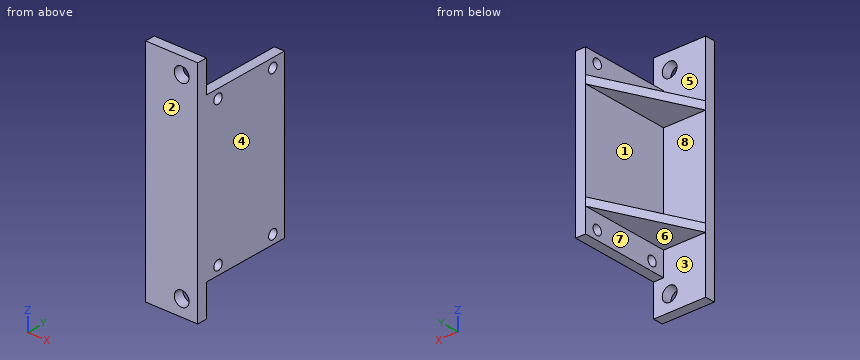
from build123d import *

# Parameters (mm, degrees)
SKETCH1_W           = 16.51
SKETCH1_H           = 71.632288028
SKETCH1_R           = 2.3495
BOSS_EXTRUDE1_DEPTH = 3.175
SKETCH2_W           = 51.312288028
SKETCH2_H           = 28.575
SKETCH2_R           = 1.524
BOSS_EXTRUDE2_DEPTH = 3.175
BOSS_EXTRUDE3_DEPTH = 2.54


with BuildPart() as part:
    # Sketch1 → Boss-Extrude1 (new body)
    with BuildSketch(Plane(origin=(0, 0, 0), x_dir=(1, 0, 0), z_dir=(0, 1, 0))):
        with Locations((-3.175, 30.736144014)):
            Rectangle(SKETCH1_W, SKETCH1_H)
        with Locations(Location((0, 61.472288028, 0), (0, 0, 270))):
            Circle(SKETCH1_R, mode=Mode.SUBTRACT)
        with Locations(Location((0, 0, 0), (0, 0, 270))):
            Circle(SKETCH1_R, mode=Mode.SUBTRACT)
    extrude(amount=BOSS_EXTRUDE1_DEPTH)

    # Sketch2 → Boss-Extrude2 (add)
    with BuildSketch(Plane(origin=(5.08, 0, 0), x_dir=(0, 0, -1), z_dir=(1, 0, 0))):
        with Locations((30.736144014, 17.4625)):
            Rectangle(SKETCH2_W, SKETCH2_H)
        with Locations((7.921390431, 7.4295)):
            Circle(SKETCH2_R, mode=Mode.SUBTRACT)
        with Locations((53.550897597, 7.4295)):
            Circle(SKETCH2_R, mode=Mode.SUBTRACT)
        with Locations((7.921390431, 27.4955)):
            Circle(SKETCH2_R, mode=Mode.SUBTRACT)
        with Locations((53.550897597, 27.4955)):
            Circle(SKETCH2_R, mode=Mode.SUBTRACT)
    extrude(amount=-BOSS_EXTRUDE2_DEPTH)

    # Sketch3 → Boss-Extrude3 (add)
    with BuildSketch(Plane(origin=(0, 0, -48.772288028), x_dir=(-1, 0, 0), z_dir=(0, 0, -1))):
        Polygon((-1.905, 31.75), (-1.905, 3.175), (11.43, 3.175), align=None)
    boss_extrude3 = extrude(amount=-BOSS_EXTRUDE3_DEPTH)

    # Mirror1: Boss-Extrude3 across plane
    add(boss_extrude3.mirror(Plane.XY.offset(-30.736144014)))


solid = part.part
The listing builds one solid part. Answer for the finished solid, in the listing's coordinates (mm). Face numbers are marked on the shaded views. A direction names the side the tool comes from. Coordinates: 2 decimals unless noted, no trailing zeros. Write each loop counter-clockwise with the first axis right and the second up, starting at its lowest first coordinate (ties: lowest second). Pieces come first, ordered by that corner, then holes. Notation, with made-up numbers: M 66,-21.75 L 93,-21.75 A17 ccw 93,7.25 Z; hole C 36,0.25 d2. An arc over 180 degrees is marked long. Put each result on its own line as item: value. Start each with the question number.
1. For a pull along Z with two mould halves and no side action, classify the marked faces 6, 7 and 8 as pulls with the +Z half, pulls with the -Z half, needs draft (parallel to the pull), parting line crosses it, or undercut.
2. Consider line 1 (Z direction, x = -7.5, y = 7); line 2 (Y direction, x = -9.25, z = -9) (3 decimals); line 3 (X direction, y = 30, z = -7) (3 decimals). Determine where each line is inside the solid, lowest interval first. Write a range as from..to.
3. A cutting plane is placed at A-A on x = 0. Write down the section's boundary in (y, z) (1 decimal).
4. A cutting plane is placed at D-D on y = 12.5. Write down the section's boundary in (x, z) (3 decimals), then the cut area to 3 significant figures.
5. A cutting plane is placed at B-B on z = 0. Write down the section's boundary in (x, y) (1 decimal), then the cut area to 3 significant figures.
6. Flat-ended cylindrical pins translate along their axes: P1, Ø6, axis at y = 20, z = -53, coming from the -X side (3 decimals); P2, Ø5, axis at x = -1.5, z = -18, coming from the +Y side (3 decimals); P3, Ø5, axis at x = -1.5, y = 20, coming from the +Z side. Find the tip coordinate at first contact, or state that the pin passes through.
7. A cutting plane is placed at C-C on x = 3.25. Count the separate pieces of the cut face and the enclosed holes in it, then the cut area to 3 significant figures.
8. Which of the six approach directions +Z, -Z, +X, -X, +Y, -Y give full straight-line access (tool end or side, diameter ignored) to the marked faces 1, 2, 3, 4 and 5?
Resolved:
1. face 6: pulls with the -Z half
1. face 7: needs draft
1. face 8: undercut
2. line 1: z = -48.77..-46.23, -15.24..-12.7
2. line 2: y = 0..3.175
2. line 3: x = 1.905..5.08
3. outline: M 0,-66.6 L 3.2,-66.6 L 3.2,-63.8 L 0,-63.8 Z; M 0,-59.1 L 3.2,-59.1 L 3.2,-48.8 L 27.7,-48.8 L 27.7,-46.2 L 3.2,-46.2 L 3.2,-15.2 L 27.7,-15.2 L 27.7,-12.7 L 3.2,-12.7 L 3.2,-2.3 L 0,-2.3 Z; M 0,2.3 L 3.2,2.3 L 3.2,5.1 L 0,5.1 Z
4. outline: M -7.078,-48.772 L 1.905,-48.772 L 1.905,-56.392 L 5.08,-56.392 L 5.08,-5.08 L 1.905,-5.08 L 1.905,-12.7 L -7.078,-12.7 L -7.078,-15.24 L 1.905,-15.24 L 1.905,-46.232 L -7.078,-46.232 Z
4. area: 209 mm2
5. outline: M -11.4,0 L -2.3,0 L -2.3,3.2 L -11.4,3.2 Z; M 2.3,0 L 5.1,0 L 5.1,3.2 L 2.3,3.2 Z
5. area: 37.5 mm2
6. P1: stops at x = 1.905
6. P2: stops at y = 3.175
6. P3: stops at z = -12.7
7. separate pieces: 1
7. enclosed holes: 4
7. area: 1,660 mm2
8. face 1: -X, +Y
8. face 2: +Z, -Z, +X, -X, -Y
8. face 3: -Z, -X, +Y
8. face 4: +Z, -Z, +X, +Y, -Y
8. face 5: +Z, -X, +Y
